Part print with two shaded views. Sizes in mm from the minimum x, y, z corner. Coordinates: 2 decimals unless noted, no trailing zeros. Write each loop counter-clockwise with the first axis right and the second up, starting at its lowest first coordinate (ties: lowest second). Pieces come first, ordered by that corner, then holes. Notation, with made-up numbers: M 13.5,85 L 38.5,85 A21 ccw 38.5,102 Z; hole C 27,-26.5 d10. An arc over 180 degrees is marked long. One line per question, with ' | ' between items. Start each with the question number.
(1) Cut at A-A (y = 15.5). Write the cut outline in (x, z), plus the area to 3 significant figures.
(2) Cut at C-C (y = 5.5). Write the cut outline in (x, z), plus the area to 3 significant figures.
(3) Cut at B-B (x = 6.5). Write the cut outline in (y, z), plus the area to 3 significant figures.
(4) Cut at D-D (z = 0.25). Write the cut outline in (x, y).
(5) Wall check: probe 1 along X at (y, z) = (17.5, 0.85); probe 2 along Y at (x, z) = (15.5, 0.7); probe 3 along X at (y, z) = (12.5, 0.8). Give the ranges that are in metal, low to high.
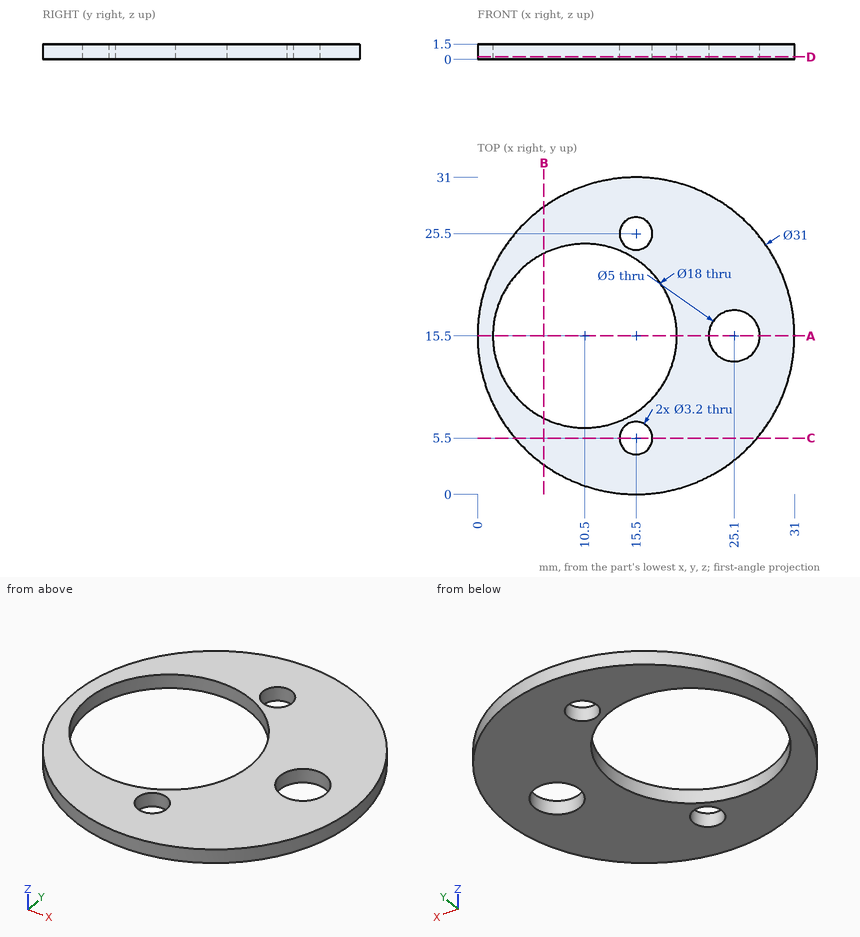
Filled in:
1) outline: M 0,0 L 1.5,0 L 1.5,1.5 L 0,1.5 Z; M 19.5,0 L 22.6,0 L 22.6,1.5 L 19.5,1.5 Z; M 27.6,0 L 31,0 L 31,1.5 L 27.6,1.5 Z | area: 12.0 mm²
2) outline: M 3.66,0 L 13.9,0 L 13.9,1.5 L 3.66,1.5 Z; M 17.1,0 L 27.34,0 L 27.34,1.5 L 17.1,1.5 Z | area: 30.7 mm²
3) outline: M 2.88,0 L 7.44,0 L 7.44,1.5 L 2.88,1.5 Z; M 23.56,0 L 28.12,0 L 28.12,1.5 L 23.56,1.5 Z | area: 13.7 mm²
4) outline: C 15.5,15.5 d31; hole C 10.5,15.5 d18; hole C 15.5,5.5 d3.2; hole C 15.5,25.5 d3.2; hole C 25.1,15.5 d5
5) probe 1: 0.13 to 1.73, 19.27 to 23.6, 26.6 to 30.87 | probe 2: 0 to 3.9, 7.1 to 8.02, 22.98 to 23.9, 27.1 to 31 | probe 3: 0.29 to 2.01, 18.99 to 30.71
